```python
from build123d import *

# Parameters (mm, degrees)
BOSS_EXTRUDE1_DEPTH = 2.521826736
SKETCH2_R           = 11.136118556
BOSS_EXTRUDE2_DEPTH = 50.8
SKETCH3_W           = 86.137031446
SKETCH3_H           = 59.748072355
BOSS_EXTRUDE3_DEPTH = 50.8
CUT_EXTRUDE1_DEPTH  = 109.100560925


with BuildPart() as part:
    # Sketch1 → Boss-Extrude1 (new body)
    with BuildSketch(Plane.XY):
        with BuildLine():
            Line((-11.136118556, 0), (-11.136118556, 25.4))
            Line((-11.136118556, 25.4), (11.136118556, 25.4))
            Line((11.136118556, 25.4), (11.136118556, 0))
            ThreePointArc((11.136118556, 0), (0, 11.136118556), (-11.136118556, 0))
        make_face()
    boss_extrude1 = extrude(amount=BOSS_EXTRUDE1_DEPTH)

    # Sketch2 → Boss-Extrude2 (add)
    with BuildSketch(Plane.XY):
        Circle(SKETCH2_R)
    extrude(amount=BOSS_EXTRUDE2_DEPTH)

    # Sketch3 → Boss-Extrude3 (add)
    with BuildSketch(Plane.XY):
        with Locations((0, 55.274036178)):
            Rectangle(SKETCH3_W, SKETCH3_H)
    extrude(amount=BOSS_EXTRUDE3_DEPTH)

    # Sketch4 → Cut-Extrude1 (cut, through all)
    with BuildSketch(Plane.XY.offset(50.8)):
        Polygon((20.431484277, 85.148072355), (20.431484277, 59.748072355), (31.75, 59.748072355), (31.75, 34.29), (-31.75, 34.29), (-31.75, 59.748072355), (-20.431484277, 59.748072355), (-20.431484277, 85.148072355), align=None)
    extrude(amount=-CUT_EXTRUDE1_DEPTH, mode=Mode.SUBTRACT)

    # Mirror1: Boss-Extrude1 across plane
    add(boss_extrude1.mirror(Plane(origin=(0, 0, 12.7), x_dir=(1, 0, 0), z_dir=(0, 0, -1))))


solid = part.part
```
The model under review builds one solid part; all positions refer to its coordinate system, in mm. A direction names the side the tool comes from. Round coordinates to 2 decimals unless told otherwise and drop trailing zeros. Order: outer loops, then holes, each group sorted by start corner. A loop starts at its lowest first (then second) coordinate and runs counter-clockwise, first axis right, second up. Notation, with made-up numbers: M -28,1 L 3,1 A8 ccw 3,8 Z; hole C -37.75,25 d9. An arc over 180 degrees is marked long. Use a Markdown table: item, result.
1) Consider section C-C (z = 42). Write out the cut boundary in (x, y).
Report:
| item | result |
|---|---|
| outline | M -43.07,25.4 L 43.07,25.4 L 43.07,85.15 L 20.43,85.15 L 20.43,59.75 L 31.75,59.75 L 31.75,34.29 L -31.75,34.29 L -31.75,59.75 L -20.43,59.75 L -20.43,85.15 L -43.07,85.15 Z; C 0,0 d22.27 |
2) Insertion check: pin 1 (1.3 mm diameter, centred on y = 8, z = 24.5, fed in from +X); pin 2 (5.5 mm diameter, centred on x = -27, z = 31, fed in from -Y); pin 3 (2 mm diameter, centred on x = 7, z = 32, fed in from +Y). Each pin has a flat end and moves straight along its axis. Give the tip position at first contact, or say it passes through.
Report:
| item | result |
|---|---|
| pin 1 | x = 11.14 |
| pin 2 | y = 25.4 |
| pin 3 | y = 34.29 |
3) Draft analysis for pull direction Z (two halves, no side actions). For faces 4 (the face through (-32, 85.148, 25)), 5 (the face through (-1, 29, 50.8)), 6 (the face through (0, 19, 2.522)), state which applies: released by +Z, released by -Z, zero draft, split by the parting line, or undercut.
Report:
| item | result |
|---|---|
| face 4 | zero draft |
| face 5 | released by +Z |
| face 6 | undercut |
4) Consider section B-B (y = 45.5). Write out the cut boundary in (x, z).
Report:
| item | result |
|---|---|
| outline | M -43.07,0 L -31.75,0 L -31.75,50.8 L -43.07,50.8 Z; M 31.75,0 L 43.07,0 L 43.07,50.8 L 31.75,50.8 Z |
5) Tool access review of faces 1 (the face through (31.75, 47, 26)), 2 (the face through (-20.431, 72, 26)), 3 (the face through (11.136, 13, 1)): name each direction out of +Z, -Z, +X, -X, +Y, -Y from which nothing blocks a thin tool from reaching the whole face with its end or side.
Report:
| item | result |
|---|---|
| face 1 | +Z, -Z |
| face 2 | +Z, -Z, +Y |
| face 3 | +Z, -Z, +X, -Y |
6) Consider section A-A (x = 25.5). Write out the cut boundary in (y, z), then the cut area to 3 significant figures.
Report:
| item | result |
|---|---|
| outline | M 25.4,0 L 34.29,0 L 34.29,50.8 L 25.4,50.8 Z; M 59.75,0 L 85.15,0 L 85.15,50.8 L 59.75,50.8 Z |
| area | 1,740 mm^2 |
7) Consider section D-D (x = 0). Write out the cut boundary in (y, z).
Report:
| item | result |
|---|---|
| outline | M -11.14,0 L 34.29,0 L 34.29,50.8 L 25.4,50.8 L 25.4,25.4 L 11.14,25.4 L 11.14,50.8 L -11.14,50.8 Z; hole M 11.14,2.52 L 25.4,2.52 L 25.4,22.88 L 11.14,22.88 Z |
8) Wall thickness on line 1 along X through (y, z) = (70.5, 23.5); line 2 along X through (y, z) = (49, 33); line 3 along Z through (x, y) = (1.5, 23.5): over which ranges is each line inside the solid? List them lowest first. Write a range as [from, to].
Report:
| item | result |
|---|---|
| line 1 | [-43.07, -20.43], [20.43, 43.07] |
| line 2 | [-43.07, -31.75], [31.75, 43.07] |
| line 3 | [0, 2.52], [22.88, 25.4] |
